```python
from build123d import *

# Parameters (mm, degrees)
F0_R     = 6.35
F1_DEPTH = 19.05
F2_W     = 25.4
F2_H     = 25.4
F3_DEPTH = 25.4


with BuildPart() as f1:
    # F0 (on Front) → F1 (new body, symmetric)
    with BuildSketch(Plane.XZ):
        with BuildLine():
            ThreePointArc((0, -12.7), (8.9802561211, -8.9802561211), (12.7, 0))
            ThreePointArc((12.7, 0), (8.9802561211, 8.9802561211), (0, 12.7))
            ThreePointArc((0, 12.7), (-8.9802561211, 8.9802561211), (-12.7, 0))
            ThreePointArc((-12.7, 0), (-8.9802561211, -8.9802561211), (0, -12.7))
        make_face()
        Circle(F0_R, mode=Mode.SUBTRACT)
        with BuildLine():
            Line((12.7, -12.7), (12.7, 0))
            ThreePointArc((12.7, 0), (8.9802561211, -8.9802561211), (0, -12.7))
            Line((0, -12.7), (12.7, -12.7))
        make_face()
        with BuildLine():
            ThreePointArc((0, 12.7), (8.9802561211, 8.9802561211), (12.7, 0))
            Line((12.7, 0), (12.7, 12.7))
            Line((12.7, 12.7), (0, 12.7))
        make_face()
        with BuildLine():
            ThreePointArc((-12.7, 0), (-8.9802561211, 8.9802561211), (0, 12.7))
            Line((0, 12.7), (-12.7, 12.7))
            Line((-12.7, 12.7), (-12.7, 0))
        make_face()
        with BuildLine():
            Line((-12.7, -12.7), (0, -12.7))
            ThreePointArc((0, -12.7), (-8.9802561211, -8.9802561211), (-12.7, 0))
            Line((-12.7, 0), (-12.7, -12.7))
        make_face()
        Polygon((12.7, -12.7), (0, -12.7), (-12.7, -12.7), (-12.7, -114.3), (0, -114.3), (12.7, -114.3), align=None)
        with BuildLine():
            Line((12.7, -127), (12.7, -114.3))
            Line((12.7, -114.3), (0, -114.3))
            ThreePointArc((0, -114.3), (8.9802561211, -118.0197438789), (12.7, -127))
        make_face()
        with BuildLine():
            Line((0, -114.3), (-12.7, -114.3))
            Line((-12.7, -114.3), (-12.7, -127))
            ThreePointArc((-12.7, -127), (-8.9802561211, -118.0197438789), (0, -114.3))
        make_face()
        with BuildLine():
            ThreePointArc((0, -139.7), (8.9802561211, -135.9802561211), (12.7, -127))
            ThreePointArc((12.7, -127), (8.9802561211, -118.0197438789), (0, -114.3))
            ThreePointArc((0, -114.3), (-8.9802561211, -118.0197438789), (-12.7, -127))
            ThreePointArc((-12.7, -127), (-8.9802561211, -135.9802561211), (0, -139.7))
        make_face()
        with Locations((0, -127)):
            Circle(F0_R, mode=Mode.SUBTRACT)
        with BuildLine():
            Line((12.7, -139.7), (12.7, -127))
            ThreePointArc((12.7, -127), (8.9802561211, -135.9802561211), (0, -139.7))
            Line((0, -139.7), (12.7, -139.7))
        make_face()
        with BuildLine():
            ThreePointArc((0, -139.7), (-8.9802561211, -135.9802561211), (-12.7, -127))
            Line((-12.7, -127), (-12.7, -139.7))
            Line((-12.7, -139.7), (0, -139.7))
        make_face()
    extrude(amount=F1_DEPTH, both=True)

    # F2 (on Right) → F3 (cut, symmetric)
    with BuildSketch(Plane.YZ):
        Rectangle(F2_W, F2_H)
        with Locations((0, -127)):
            Rectangle(F2_W, F2_H)
    extrude(amount=F3_DEPTH, both=True, mode=Mode.SUBTRACT)


solid = f1.part
```
Can you work these out from the model? Positions are in its coordinate system, mm. A direction names the side the tool comes from. Give positions to 0.01 mm unless a question says otherwise; leave off trailing zeros. Loops run counter-clockwise (first coordinate to the right, second up) from the corner with the lowest first, then second, coordinate; pieces in that order, holes last. Notation, with made-up numbers: M -4,25.5 L 36,25.5 A22 cw 36,46.5 Z; hole C -24,6 d1. An arc over 180 degrees is marked long. Use CSV: the item, a comma, the result in double quotes. Start each with the question number.
1. On a 3-axis mill with a long thin cutter (end or side, diameter ignored), from which of +Z, -Z, +X, -X, +Y, -Y can I reach the whole of each face in a straight line? I mean faces 1 (the face through (-6, -12.7, -3)), 2 (the face through (6, 12.7, -130)), 3 (the face through (0, -19.05, -62)). Say none if no direction works.
2. Imagine slicing it at C-C, the plane y = 14. Write out the boundary of the cut face in (x, z), plus the area to 3 significant figures.
3. Imagine slicing it at D-D, the plane z = -127. Write out the boundary of the cut face in (x, y), plus the area to 3 significant figures.
4. If I drill on L1, parallel to Z at x = 0, y = 17.25; L2, parallel to Y at x = 5.5, z = -122; L3, parallel to X at y = 17.25, z = 0, over which ranges is the centre line in solid material (lowest first)?
5. Imagine slicing it at A-A, the plane x = 0. Write out the boundary of the cut face in (y, z).
6. If we mould it in two halves opening along X, with no side actions, what happens to faces 4 (the face through (12.7, 0, -65)), 5 (the face through (3.414, -15.831, -121.646)), 6 (the face through (0, 0, -114.3))? For each: released by +X, released by -X, zero draft, split by the parting line, or undercut.
7. For P1, Ø7.5, axis at x = 1, z = -122, coming from the +Y side; P2, Ø1.5, axis at x = 8, y = -4, coming from the +Z side; P3, Ø7.5, axis at x = 1.5, z = 1, coming from the +Y side; P4, Ø1, axis at x = 10, y = 0.5, coming from the -Z side, each with a flat end and sliding along its axis, tell me the tip position at first contact or that it passes through.
8. Imagine slicing it at B-B, the plane z = -9.5. Write out the boundary of the cut face in (x, y), plus the area to 3 significant figures.
Response values:
1,face 1,"+Z, +X, -X"
1,face 2,"-Z, +X, -X"
1,face 3,"+Z, -Z, +X, -X, -Y"
2,outline,"M -12.7,-139.7 L 12.7,-139.7 L 12.7,12.7 L -12.7,12.7 Z; hole C 0,-127 d12.7; hole C 0,0 d12.7"
2,area,"3,620 mm^2"
3,outline,"M -12.7,-19.05 L -6.35,-19.05 L -6.35,-12.7 L -12.7,-12.7 Z; M -12.7,12.7 L -6.35,12.7 L -6.35,19.05 L -12.7,19.05 Z; M 6.35,-19.05 L 12.7,-19.05 L 12.7,-12.7 L 6.35,-12.7 Z; M 6.35,12.7 L 12.7,12.7 L 12.7,19.05 L 6.35,19.05 Z"
3,area,"161 mm^2"
4,L1,"-139.7 to -133.35, -120.65 to -6.35, 6.35 to 12.7"
4,L2,"-19.05 to -12.7, 12.7 to 19.05"
4,L3,"-12.7 to -6.35, 6.35 to 12.7"
5,outline,"M -19.05,-139.7 L -12.7,-139.7 L -12.7,-133.35 L -19.05,-133.35 Z; M -19.05,-120.65 L -12.7,-120.65 L -12.7,-114.3 L 12.7,-114.3 L 12.7,-120.65 L 19.05,-120.65 L 19.05,-6.35 L 12.7,-6.35 L 12.7,-12.7 L -12.7,-12.7 L -12.7,-6.35 L -19.05,-6.35 Z; M -19.05,6.35 L -12.7,6.35 L -12.7,12.7 L -19.05,12.7 Z; M 12.7,-139.7 L 19.05,-139.7 L 19.05,-133.35 L 12.7,-133.35 Z; M 12.7,6.35 L 19.05,6.35 L 19.05,12.7 L 12.7,12.7 Z"
6,face 4,"released by +X"
6,face 5,"undercut"
6,face 6,"zero draft"
7,P1,"y = 19.05"
7,P2,"z = -12.7"
7,P3,"through"
7,P4,"z = -114.3"
8,outline,"M -12.7,-19.05 L 12.7,-19.05 L 12.7,-12.7 L -12.7,-12.7 Z; M -12.7,12.7 L 12.7,12.7 L 12.7,19.05 L -12.7,19.05 Z"
8,area,"323 mm^2"
